Read the model definition and answer for the solid it produces. Units are mm, in the model's axes. Coordinates: 2 decimals unless noted, no trailing zeros. Loops run counter-clockwise (first coordinate to the right, second up) from the corner with the lowest first, then second, coordinate; pieces in that order, holes last.
Autodesk Fusion 360 part; units mm, degrees
sketch "Sketch1" plane through (0, 0, 0) normal (0, 1, 0) x (1, 0, 0)
  line L0 (0, 0) -> (4, 0)
  line L1 (4, 0) -> (4, -4)
  line L2 (4, -4) -> (0, -4)
  line L3 (0, -4) -> (0, 0)
  circle A0 centre (2, -2) radius 0.8
  dimension "d1" = 4
  dimension "d2" = 4
  dimension "BORE" = 1.6
  dimension "d4" = 2
  dimension "d5" = 2
extrude "Extrude1" add sketch "Sketch1" along normal blind 16
chamfer "Chamfer1" distance 1 angle 45 4 edges at (4, 8, 4) (0, 8, 4) (0, 8, 0) (4, 8, 0)
Q1. A cutting plane is placed at D-D (x = 3.65). Give the vertices of the cut face in (y, z).
Findings below:
outline: (0, 0.65) - (16, 0.65) - (16, 3.35) - (0, 3.35) - close
Q2. A cutting plane is placed at C-C (y = 6). Give the vertices of the cut face in (x, z), then the cut area to 3 significant figures.
Findings below:
outline: (0, 1) - (1, 0) - (3, 0) - (4, 1) - (4, 3) - (3, 4) - (1, 4) - (0, 3) - close; hole circle Ø1.6 at (2, 2)
area: 12.0 mm2
Q3. Determine the mould class of faces 1 (the face through (3.5, 7.9, 3.5)), 2 (the face through (0.5, 8.1, 0.5)), 3 (the face through (2.739, 7.888, 1.694)), 4 (the face through (2, 8, 4)) for opening direction X: +X half, -X half, draft (parallel to the pull), parting line (faces both ways), or undercut.
Findings below:
face 1: +X half
face 2: -X half
face 3: undercut
face 4: draft
Q4. A cutting plane is placed at A-A (x = 2). Give the vertices of the cut face in (y, z), then the cut area to 3 significant figures.
Findings below:
outline: (0, 0) - (16, 0) - (16, 1.2) - (0, 1.2) - close; (0, 2.8) - (16, 2.8) - (16, 4) - (0, 4) - close
area: 38.4 mm2
Q5. A cutting plane is placed at B-B (z = 2). Give the vertices of the cut face in (x, y).
Findings below:
outline: (0, 0) - (1.2, 0) - (1.2, 16) - (0, 16) - close; (2.8, 0) - (4, 0) - (4, 16) - (2.8, 16) - close
Q6. Straight lines are drawn through the part: probe 1 along Z at (x, y) = (2, 5.25); probe 2 along X at (y, z) = (5.25, 1.4). For each, find the intervals that lie inside material, in ascending order.
Findings below:
probe 1: z = 0 to 1.2, 2.8 to 4
probe 2: x = 0 to 1.47, 2.53 to 4
